Part model, mm, in its own coordinate system. A direction names the side the tool comes from. Give positions to 0.01 mm unless a question says otherwise; leave off trailing zeros. Order: outer loops, then holes, each group sorted by start corner. A loop starts at its lowest first (then second) coordinate and runs counter-clockwise, first axis right, second up. Notation, with made-up numbers: M 8.5,-32 L 64.5,-32 A38 ccw 64.5,6 Z; hole C -26,80.5 d2. An arc over 180 degrees is marked long. Return JSON: item names as keys, results as strings.
from build123d import *

# Parameters (mm, degrees)
Y_KSEKLIK_EKSTR_ZYON1_DEPTH = 25
IZIM2_R                     = 2
KES_EKSTR_ZYON1_DEPTH       = 25
IZIM3_R                     = 3.5
IZIM3_W                     = 8
IZIM3_H                     = 30
KES_EKSTR_ZYON2_DEPTH       = 10
IZIM4_R                     = 1.5
KES_EKSTR_ZYON3_DEPTH       = 10
DAIRESEL_KAPLAMA2_COUNT     = 6
CUT_EXTRUDE8_DEPTH          = 7.5
RADYUS1_R                   = 4


with BuildPart() as part:
    # Çizim1 → Yükseklik-Ekstrüzyon1 (new body)
    with BuildSketch(Plane.XY):
        Polygon((-2.5, 69), (-12.5, 69), (-12.5, 111), (-7.5, 111), (-7.5, 80), (7.5, 80), (7.5, 111), (12.5, 111), (12.5, 69), (2.5, 69), (2.5, -69), (-2.5, -69), align=None)
    extrude(amount=Y_KSEKLIK_EKSTR_ZYON1_DEPTH)

    # Çizim2 → Kes-Ekstrüzyon1 (cut)
    with BuildSketch(Plane.ZY.offset(12.5)):
        with Locations((12.5, 98.5)):
            Circle(IZIM2_R)
    extrude(amount=-KES_EKSTR_ZYON1_DEPTH, mode=Mode.SUBTRACT)

    # Çizim3 → Kes-Ekstrüzyon2 (cut)
    with BuildSketch(Plane.ZY.offset(2.5)):
        with Locations((12.5, -54)):
            Circle(IZIM3_R)
        with Locations((12.5, 41)):
            Rectangle(IZIM3_W, IZIM3_H)
        with Locations((12.5, -14)):
            Rectangle(IZIM3_W, IZIM3_H)
    extrude(amount=-KES_EKSTR_ZYON2_DEPTH, mode=Mode.SUBTRACT)

    # Çizim4 → Kes-Ekstrüzyon3 (cut)
    with BuildSketch(Plane.ZY.offset(2.5)):
        with Locations((12.5, -44.5)):
            Circle(IZIM4_R)
    kes_ekstr_zyon3 = extrude(amount=-KES_EKSTR_ZYON3_DEPTH, mode=Mode.SUBTRACT)

    # Dairesel Kaplama2: Kes-Ekstrüzyon3 ×6 about axis
    dairesel_kaplama2_axis = Axis((0, -54, 12.5), (1, 0, 0))
    for i in range(1, DAIRESEL_KAPLAMA2_COUNT):
        add(kes_ekstr_zyon3.rotate(dairesel_kaplama2_axis, i * 360 / DAIRESEL_KAPLAMA2_COUNT), mode=Mode.SUBTRACT)

    # Sketch2 → Cut-Extrude8 (cut, symmetric)
    with BuildSketch(Plane(origin=(0, 0, 0), x_dir=(0, 0, -1), z_dir=(1, 0, 0))):
        Polygon((-12.5, 84), (-25.5, 72), (-25.5, 86), (0.5, 86), (0.5, 72), align=None)
    extrude(amount=CUT_EXTRUDE8_DEPTH, both=True, mode=Mode.SUBTRACT)

    # Radyus1
    radyus1_edges = [part.edges().sort_by_distance(p)[0] for p in [
        (-10, 111, 25),
        (10, 111, 25),
        (10, 111, 0),
        (-10, 111, 0),
        (0, 26, 16.5),
        (0, 56, 16.5),
        (0, 26, 8.5),
        (0, 56, 8.5),
        (0, -29, 16.5),
        (0, -29, 8.5),
        (0, 1, 16.5),
        (0, 1, 8.5),
        (0, -69, 25),
        (0, -69, 0),
        (0, 80, 16.833333333),
        (0, 80, 8.166666667),
        (12.5, 69, 12.5),
        (-12.5, 69, 12.5),
    ]]
    fillet(radyus1_edges, radius=RADYUS1_R - 0.0001)  # a hair under: the kernel refuses the full size


solid = part.part
Q1. 3-axis set-ups, long thin cutter, end or side, ignore diameter. For faces 1 (the flat face through (2.5, 1, 10)), 2 (the cylindrical face through (-0.035, -67.797, 23.859)), 3 (the flat face through (0, 41, 16.5)): which of +Z, -Z, +X, -X, +Y, -Y reach the whole face in a straight line?
Established:
{"face 1": "+Z, -Z, +X, -Y", "face 2": "+Z, +X, -X, -Y", "face 3": "+X, -X"}
Q2. Pin check, flat tips, straight feed: pin 1 (1.5 mm diameter, centred on x = -5.5, z = 20.5, fed in from +Y); pin 2 (3 mm diameter, centred on x = -5, y = 79.5, fed in from -Z); pin 3 (5 mm diameter, centred on y = -63.5, z = 12.5, fed in from -X). Stop position of each tip, or through.
Established:
{"pin 1": "stops at y = 77.31", "pin 2": "stops at z = 6", "pin 3": "stops at x = -2.5"}
Q3. Band-saw the part on A-A (y = -63.5). Give the cut face in (x, z).
Established:
{"outline": "M -2.5,0 L 2.5,0 L 2.5,11 L -2.5,11 Z; M -2.5,14 L 2.5,14 L 2.5,25 L -2.5,25 Z"}
Q4. Band-saw the part on B-B (y = 98.5). Give the cut face in (x, z).
Established:
{"outline": "M -12.5,0 L -7.5,0 L -7.5,10.5 L -12.5,10.5 Z; M -12.5,14.5 L -7.5,14.5 L -7.5,25 L -12.5,25 Z; M 7.5,0 L 12.5,0 L 12.5,10.5 L 7.5,10.5 Z; M 7.5,14.5 L 12.5,14.5 L 12.5,25 L 7.5,25 Z"}
Q5. Band-saw the part on C-C (x = -1). Give the number of separate pieces and of enclosed holes in the cut face, then the cut area to 3 significant figures.
Established:
{"separate pieces": "1", "enclosed holes": "9", "area": "3,120 mm²"}
Q6. Probe line 1 along Y through (x, z) = (-9, 12.25); line 2 along Y through (x, z) = (0.5, 3.25); line 3 along X through (y, z) = (92.5, 8). List the from-to ranges inside material, lowest first.
Established:
{"line 1": "y = 69.03 to 96.52, 100.48 to 111", "line 2": "y = -68.93 to -59.85, -57.65 to -50.35, -48.15 to 75.46", "line 3": "x = -12.5 to -7.5, 7.5 to 12.5"}
Q7. Two-plate mould, pull along X, no slides. Class faces 4 (the flat face through (-7.5, 96, 12)), 5 (the cylindrical face through (11.297, 70.141, 12.675)), 6 (the flat face through (-2.5, -1, 18)), 7 (the cylindrical face through (0.035, 54.797, 15.359)): +X half, -X half, draft (parallel to the pull), parting line (faces both ways), or undercut.
Established:
{"face 4": "undercut", "face 5": "+X half", "face 6": "-X half", "face 7": "draft"}
Q8. Band-saw the part on D-D (y = 40.5). Give the cut face in (x, z).
Established:
{"outline": "M -2.5,0 L 2.5,0 L 2.5,8.5 L -2.5,8.5 Z; M -2.5,16.5 L 2.5,16.5 L 2.5,25 L -2.5,25 Z"}
